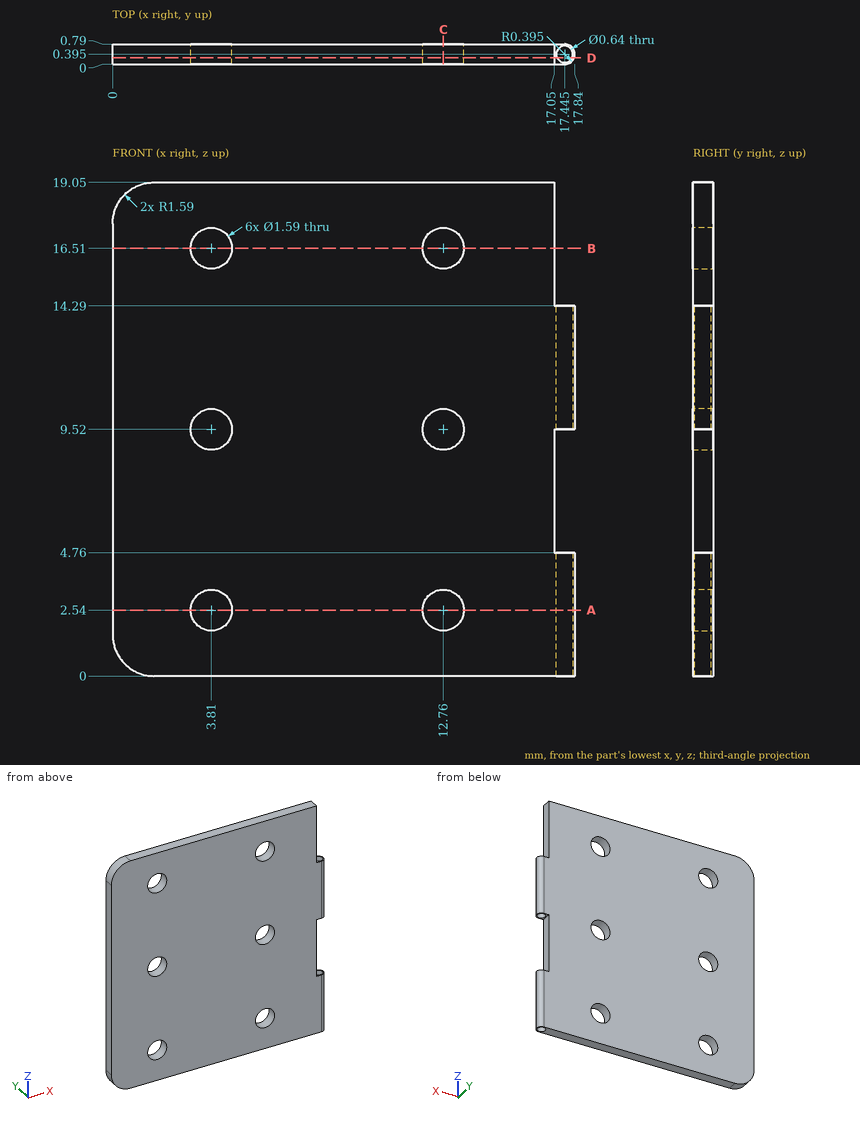
Check sheet for the drawn part. Datum: minimum x, y, z corner. Units: mm. Give positions to 0.01 mm unless a question says otherwise; leave off trailing zeros. Loops run counter-clockwise (first coordinate to the right, second up) from the corner with the lowest first, then second, coordinate; pieces in that order, holes last.
1) Sectioned sample at D-D, the plane y = 0.25. Count the separate pieces of the cut face and the enclosed holes in it, then the cut area to 3 significant figures.
2) Thickness scan on line 1 along Z through (x, y) = (3.75, 0.45); line 2 along Z through (x, y) = (4, 0.45); line 3 along X through (y, z) = (0.6, 6.5). Record the ranges inside material, lowest first.
3) Sectioned sample at A-A, the plane z = 2.54. Enter the section's corners in (x, y) (3 decimals), then the cut area to 3 significant figures.
4) Sectioned sample at C-C, the plane x = 12.76. Enter the section's corners in (y, z) (3 decimals).
5) Sectioned sample at B-B, the plane z = 16.51. Enter the section's corners in (x, y) (3 decimals).
Answers:
1. separate pieces: 3
1. enclosed holes: 6
1. area: 314 mm2
2. line 1: z = 0 to 1.75, 3.33 to 8.73, 10.31 to 15.72, 17.3 to 19.05
2. line 2: z = 0 to 1.77, 3.31 to 8.75, 10.29 to 15.74, 17.28 to 19.05
2. line 3: x = 0 to 17.05
3. outline: (0, 0) - (3.015, 0) - (3.015, 0.79) - (0, 0.79) - close; (4.605, 0) - (11.965, 0) - (11.965, 0.79) - (4.605, 0.79) - close; (13.555, 0) - (17.445, 0) arc R0.395 ccw to (17.445, 0.79) - (13.555, 0.79) - close; hole circle Ø0.64 at (17.445, 0.395)
3. area: 11.2 mm2
4. outline: (0, 0) - (0.79, 0) - (0.79, 1.745) - (0, 1.745) - close; (0, 3.335) - (0.79, 3.335) - (0.79, 8.725) - (0, 8.725) - close; (0, 10.315) - (0.79, 10.315) - (0.79, 15.715) - (0, 15.715) - close; (0, 17.305) - (0.79, 17.305) - (0.79, 19.05) - (0, 19.05) - close
5. outline: (0, 0) - (3.015, 0) - (3.015, 0.79) - (0, 0.79) - close; (4.605, 0) - (11.965, 0) - (11.965, 0.79) - (4.605, 0.79) - close; (13.555, 0) - (17.05, 0) - (17.05, 0.79) - (13.555, 0.79) - close
